The drawing under review shows one solid part. Ordinate dimensions are in mm from its lowest x, y, z. Coordinates: 2 decimals unless noted, no trailing zeros. Order: outer loops, then holes, each group sorted by start corner. A loop starts at its lowest first (then second) coordinate and runs counter-clockwise, first axis right, second up. Notation, with made-up numbers: (27.25, 35) -> (57.25, 35) arc R29 ccw to (57.25, 56) -> close; hole circle Ø11 at (83, -21.75). An arc over 180 degrees is marked (long way). Write item = value, one per line.
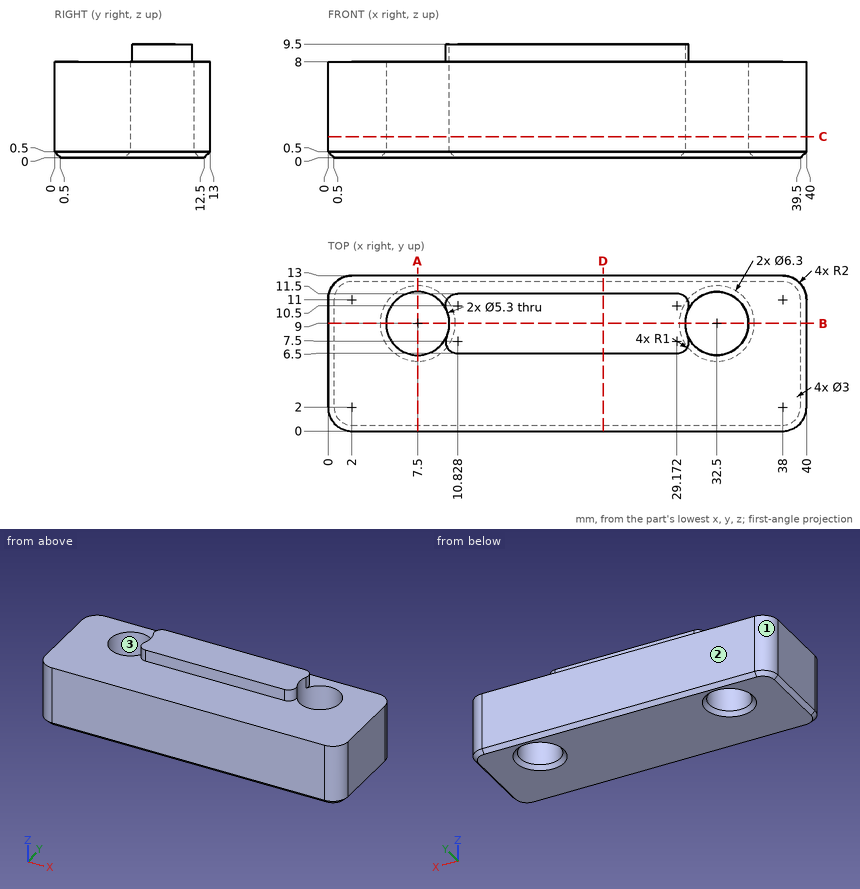
(1) For L1, parallel to Y at x = 7.5, z = 5.25; L2, parallel to X at y = 8.5, z = 1.25; L3, parallel to X at y = 10, z = 2.5 (1 decimal), list the stretches that pass through material, from the lowest coordinate up.
Report:
L1 = 0 to 6.35, 11.65 to 13
L2 = 0 to 4.9, 10.1 to 29.9, 35.1 to 40
L3 = 0 to 5, 10 to 30, 35 to 40
(2) We need section D-D (x = 23). Write out the cut boundary in (y, z), and give its area (3 significant figures).
Report:
outline = (0, 0.5) -> (0.5, 0) -> (12.5, 0) -> (13, 0.5) -> (13, 8) -> (11.5, 8) -> (11.5, 9.5) -> (6.5, 9.5) -> (6.5, 8) -> (0, 8) -> close
area = 111 mm²
(3) We need section A-A (x = 7.5). Write out the cut boundary in (y, z).
Report:
outline = (0, 0.5) -> (0.5, 0) -> (5.85, 0) -> (6.35, 0.5) -> (6.35, 8) -> (0, 8) -> close; (11.65, 0.5) -> (12.15, 0) -> (12.5, 0) -> (13, 0.5) -> (13, 8) -> (11.65, 8) -> close
(4) The part is to be moulded in two halves that separate along X. For the marked faces 1, 2 and 3, say which applies: released by +X, released by -X, zero draft, split by the parting line, or undercut.
Report:
face_1 = released by -X
face_2 = zero draft
face_3 = undercut
(5) Insertion check: pin 1 (0.8 mm diameter, centred on x = 16.5, z = 9, fed in from +Y); pin 2 (0.8 mm diameter, centred on x = 23.5, z = 9, fed in from -Y). Each pin has a flat end and moves straight along its axis. Give the tip position at first contact, or say it passes through.
Report:
pin_1 = 11.5
pin_2 = 6.5
(6) We need section C-C (z = 1.75). Write out the cut boundary in (x, y).
Report:
outline = (0, 2) arc R2 ccw to (2, 0) -> (38, 0) arc R2 ccw to (40, 2) -> (40, 11) arc R2 ccw to (38, 13) -> (2, 13) arc R2 ccw to (0, 11) -> close; hole circle Ø5.3 at (7.5, 9); hole circle Ø5.3 at (32.5, 9)
(7) We need section B-B (y = 9). Write out the cut boundary in (x, z).
Report:
outline = (0, 0.5) -> (0.5, 0) -> (4.35, 0) -> (4.85, 0.5) -> (4.85, 8) -> (0, 8) -> close; (10.15, 0.5) -> (10.65, 0) -> (29.35, 0) -> (29.85, 0.5) -> (29.85, 9.5) -> (10.15, 9.5) -> close; (35.15, 0.5) -> (35.65, 0) -> (39.5, 0) -> (40, 0.5) -> (40, 8) -> (35.15, 8) -> close
